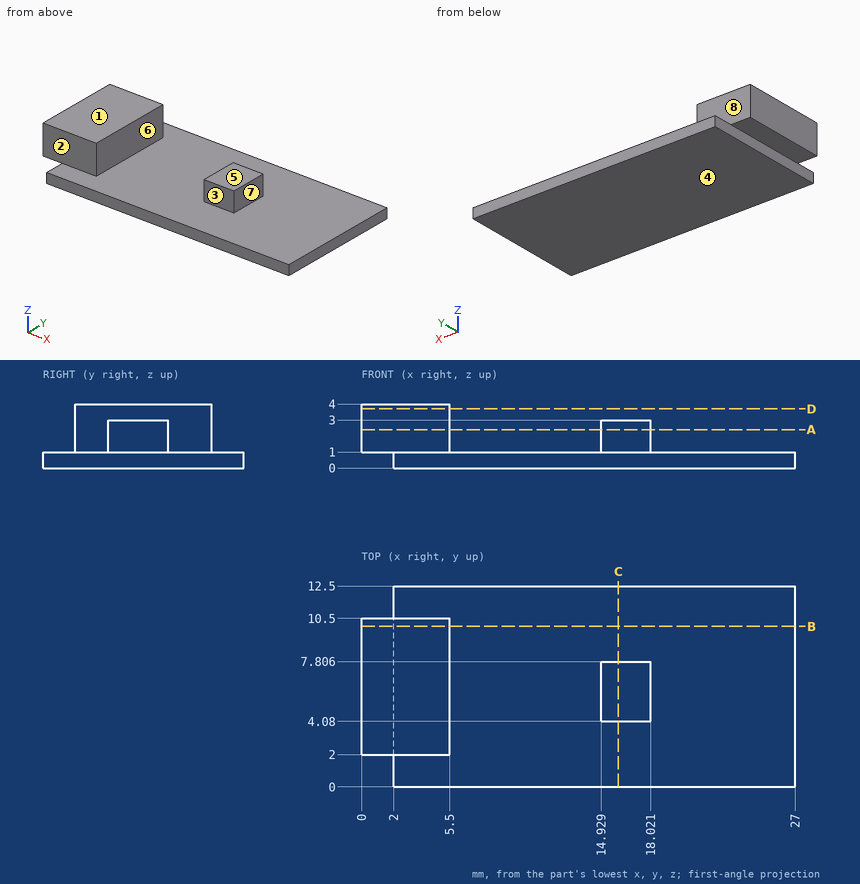
The drawing under review shows one solid part. Ordinate dimensions are in mm from its lowest x, y, z. A direction names the side the tool comes from. Coordinates: 2 decimals unless noted, no trailing zeros. Write each loop counter-clockwise with the first axis right and the second up, starting at its lowest first coordinate (ties: lowest second). Pieces come first, ordered by that corner, then holes. Notation, with made-up numbers: (-29, 23) - (28, 23) arc R28 ccw to (28, 51) - close; hole circle Ø5 at (16, -14.75). An arc over 180 degrees is marked (long way). Answer as CSV lines item,"result".
(1) We need section C-C (x = 16). Give the boundary of the cut face in (y, z) (1 decimal).
Data:
outline,"(0, 0) - (12.5, 0) - (12.5, 1) - (7.8, 1) - (7.8, 3) - (4.1, 3) - (4.1, 1) - (0, 1) - close"
(2) For line 1 along Z through (x, y) = (20, 1); line 2 along Y through (x, z) = (5, 1.2); line 3 along X through (y, z) = (4.5, 2.8), list the stretches that pass through material, from the lowest coordinate up. Write a range as [from, to].
Data:
line 1,"z = [0, 1]"
line 2,"y = [2, 10.5]"
line 3,"x = [0, 5.5], [14.93, 18.02]"
(3) Mouldability with a two-part tool opening along X and no side actions: class the marked faces 6, 7 and 8 as pulls with the +X half, pulls with the -X half, needs draft (parallel to the pull), parting line crosses it, or undercut.
Data:
face 6,"undercut"
face 7,"pulls with the +X half"
face 8,"needs draft"
(4) We need section D-D (z = 3.7). Give the boundary of the cut face in (x, y).
Data:
outline,"(0, 2) - (5.5, 2) - (5.5, 10.5) - (0, 10.5) - close"
(5) We need section B-B (y = 10). Give the boundary of the cut face in (x, z).
Data:
outline,"(0, 1) - (2, 1) - (2, 0) - (27, 0) - (27, 1) - (5.5, 1) - (5.5, 4) - (0, 4) - close"
(6) Tool access review of the marked faces 1, 2, 3, 4 and 5: name each direction out of +Z, -Z, +X, -X, +Y, -Y from which nothing blocks a thin tool from reaching the whole face with its end or side.
Data:
face 1,"+Z, +X, -X, +Y, -Y"
face 2,"+Z, +X, -X, -Y"
face 3,"+Z, +X, -Y"
face 4,"-Z, +X, -X, +Y, -Y"
face 5,"+Z, +X, +Y, -Y"
(7) Clearance check with flat-ended pins moving along their axes: pin 1 Ø2 at (x, z) = (16, 2.5) entering from +Y; pin 2 Ø6 at (x, y) = (11.5, 6.5) entering from +Z; pin 3 Ø0.5 at (y, z) = (5, 0.5) entering from -X. State where each tip first meets the part, or that it passes through.
Data:
pin 1,"stops at y = 7.81"
pin 2,"stops at z = 1"
pin 3,"stops at x = 2"
(8) We need section A-A (z = 2.4). Give the boundary of the cut face in (x, y) (1 decimal).
Data:
outline,"(0, 2) - (5.5, 2) - (5.5, 10.5) - (0, 10.5) - close; (14.9, 4.1) - (18, 4.1) - (18, 7.8) - (14.9, 7.8) - close"
